Check sheet for the drawn part. Datum: minimum x, y, z corner. Units: mm. A direction names the side the tool comes from. Give positions to 0.01 mm unless a question says otherwise; leave off trailing zeros. Order: outer loops, then holes, each group sorted by start corner. A loop starts at its lowest first (then second) coordinate and runs counter-clockwise, first axis right, second up.
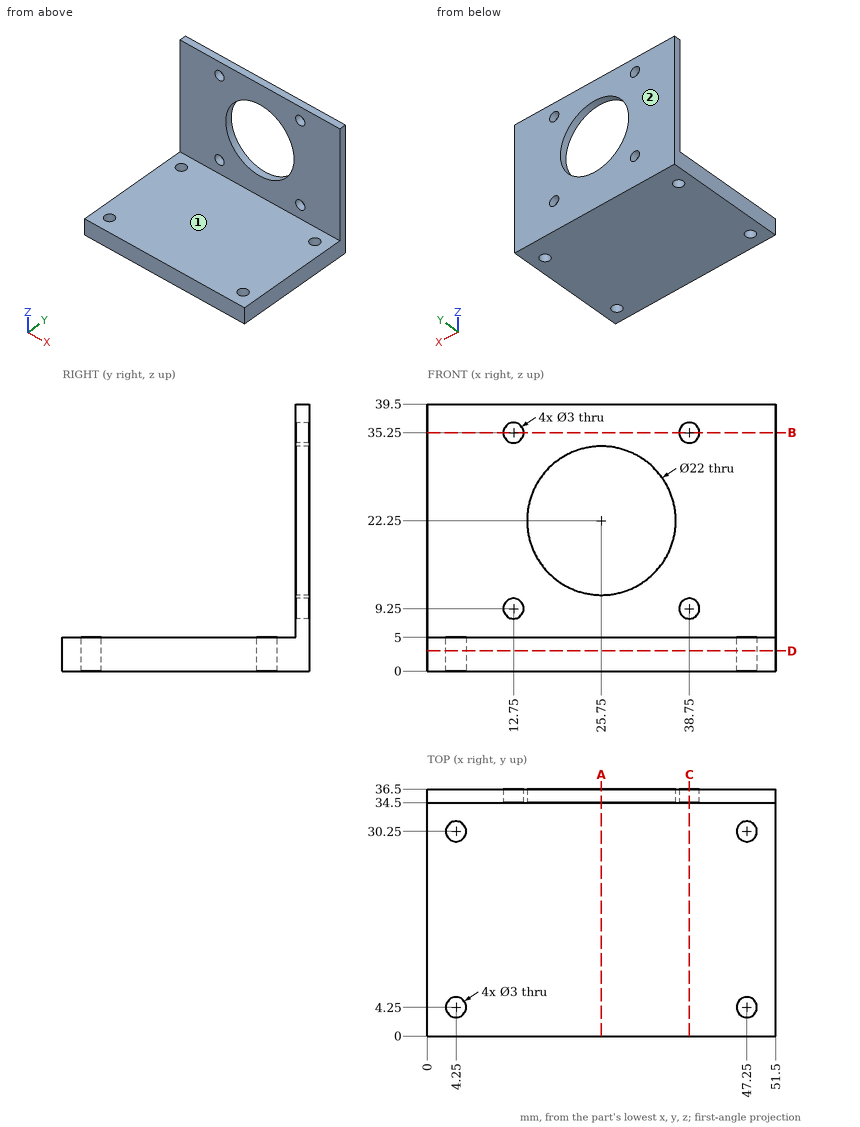
(1) Section check A-A, the plane x = 25.75. Enter the section's corners in (y, z).
Solved:
outline: (0, 0) - (36.5, 0) - (36.5, 11.25) - (34.5, 11.25) - (34.5, 5) - (0, 5) - close; (34.5, 33.25) - (36.5, 33.25) - (36.5, 39.5) - (34.5, 39.5) - close
(2) Go/stop test with flat-tipped pins: pin 1 (5 mm diameter, centred on x = 12.75, z = 9.25, fed in from -Y); pin 2 (10.5 mm diameter, centred on x = 28.5, y = 22.5, fed in from +Z). Record where each tip stops, or that it passes through.
Solved:
pin 1: stops at y = 34.5
pin 2: stops at z = 5
(3) Scan lines: line 1 (Z direction, x = 38.75, y = 35.2); line 2 (Y direction, x = 4.25, z = 3.15); line 3 (Y direction, x = 41, z = 11.5). Record each from-to range of solid material in increasing order.
Solved:
line 1: z = 0 to 7.75, 10.75 to 33.75, 36.75 to 39.5
line 2: y = 0 to 2.75, 5.75 to 28.75, 31.75 to 36.5
line 3: y = 34.5 to 36.5
(4) Section check B-B, the plane z = 35.25. Enter the section's corners in (x, y).
Solved:
outline: (0, 34.5) - (11.25, 34.5) - (11.25, 36.5) - (0, 36.5) - close; (14.25, 34.5) - (37.25, 34.5) - (37.25, 36.5) - (14.25, 36.5) - close; (40.25, 34.5) - (51.5, 34.5) - (51.5, 36.5) - (40.25, 36.5) - close
(5) Section check D-D, the plane z = 3. Enter the section's corners in (x, y).
Solved:
outline: (0, 0) - (51.5, 0) - (51.5, 36.5) - (0, 36.5) - close; hole circle Ø3 at (4.25, 4.25); hole circle Ø3 at (4.25, 30.25); hole circle Ø3 at (47.25, 4.25); hole circle Ø3 at (47.25, 30.25)
(6) Set-up check for the marked faces 1 and 2: record each of +Z, -Z, +X, -X, +Y, -Y from which the full face is reachable in a straight line by a thin tool's end or side.
Solved:
face 1: +Z, +X, -X, -Y
face 2: +Z, -Z, +X, -X, +Y
(7) Section check C-C, the plane x = 38.75. Enter the section's corners in (y, z).
Solved:
outline: (0, 0) - (36.5, 0) - (36.5, 7.75) - (34.5, 7.75) - (34.5, 5) - (0, 5) - close; (34.5, 10.75) - (36.5, 10.75) - (36.5, 33.75) - (34.5, 33.75) - close; (34.5, 36.75) - (36.5, 36.75) - (36.5, 39.5) - (34.5, 39.5) - close
